Geometry check sheet. Reference: the model listing, model coordinates, mm. A direction names the side the tool comes from. Coordinates: 2 decimals unless noted, no trailing zeros. Write each loop counter-clockwise with the first axis right and the second up, starting at its lowest first coordinate (ties: lowest second). Pieces come first, ordered by that corner, then holes. Notation, with made-up numbers: (45, 76.25) -> (70, 76.25) arc R7 cw to (70, 86.25) -> close; hole circle Ø7 at (-33.75, -22.75). An arc over 180 degrees is marked (long way). Answer in a Markdown table with one row per item. Add a question column.
1. Cross-section at A-A on x = -64. Record the cut outline in (y, z).
2. Cross-section at D-D on x = 0. Record the cut outline in (y, z), and give its area (3 significant figures).
3. Depth check by flat-ended pin: P1, Ø2, axis at x = 3.5, z = -30.5, coming from the +Y side; P2, Ø15.5, axis at y = 13.5, z = -12.5, coming from the +X side; P3, Ø25, axis at y = 18, z = 13.5, coming from the -X side. Enter the tip coordinate at first touch or a pass-through.
4. Mould release check, pull along Z, two halves, no side actions. Record for faces 5 (the cylindrical face through (-64, 38, 27)), 6 (the flat face through (0, -16, 59.5)), 7 (the cylindrical face through (49.783, 37.147, -0.7)): pulls with the +Z half, pulls with the -Z half, needs draft (parallel to the pull), parting line crosses it, or undercut.
5. Scan lines: L1, parallel to X at y = 34, z = -49; L2, parallel to X at y = 37.55, z = -30; L3, parallel to X at y = 37.65, z = -30. Record each from-to range of solid material in increasing order. Write a range as from..to.
6. Cross-section at C-C on y = 31.5. Record the cut outline in (x, z).
7. Cross-section at B-B on z = -30. Record the cut outline in (x, y), and give its area (3 significant figures).
8. Set-up check for faces 1 (the flat face through (48.5, 19, 1)), 2 (the flat face through (0, -16, 58)), 3 (the flat face through (-50, 18, -1)), 4 (the flat face through (10, -9.2, 58.2)): record each of +Z, -Z, +X, -X, +Y, -Y from which the full face is reachable in a straight line by a thin tool's end or side.
```python
from build123d import *

# Parameters (mm, degrees)
SKETCH1_R                      = 5
BASE_FLANGE1_DEPTH             = 1.5
EDGE_FLANGE1_STRIP_W           = 12
EDGE_FLANGE1_STRIP_H           = 1.5
EDGE_FLANGE1_STRIP_CUT_DEPTH   = 100
EDGE_FLANGE1_STRIP_2_W         = 12
EDGE_FLANGE1_STRIP_2_H         = 1.5
EDGE_FLANGE1_STRIP_CUT_2_DEPTH = 100
EDGE_FLANGE1_DEPTH             = 100
EDGE_FLANGE1_BEND_DEPTH        = 100
EDGE_FLANGE2_STRIP_W           = 12
EDGE_FLANGE2_STRIP_H           = 1.5
EDGE_FLANGE2_STRIP_CUT_DEPTH   = 100
EDGE_FLANGE2_STRIP_2_W         = 12
EDGE_FLANGE2_STRIP_2_H         = 1.5
EDGE_FLANGE2_STRIP_CUT_2_DEPTH = 100
EDGE_FLANGE2_DEPTH             = 100
EDGE_FLANGE2_BEND_DEPTH        = 100
SKETCHED_START                 = 58.9178
SKETCHED_BEND1_OUTLINE_W       = 20
SKETCHED_BEND1_OUTLINE_H       = 1.5
SKETCHED_BEND1_DEPTH           = 32.0822
SKETCHED_START_2               = 56.266894772
SKETCHED_BEND1_2_OUTLINE_R     = 5
SKETCHED_BEND1_2_DEPTH         = 3.233105228
SKETCHED_START_3               = -10
SKETCHED_BEND1_3_DEPTH         = 20
SKETCHED_BEND1_4_DEPTH         = 20
SKETCH21_R                     = 3
CUT_EXTRUDE1_DEPTH             = 10


with BuildPart() as part:
    # Base-Flange1: sheet metal written as solids
    # Sketch1 → Base-Flange1 (new body)
    with BuildSketch(Plane(origin=(0, 0, 0), x_dir=(1, 0, 0), z_dir=(0, 1, 0))):
        with BuildLine():
            Line((10, 50), (10, 80))
            ThreePointArc((10, 80), (0, 90), (-10, 80))
            Line((-10, 80), (-10, 50))
            Line((-10, 50), (-50, 50))
            Line((-50, 50), (-50, -50))
            Line((-50, -50), (-10, -50))
            Line((-10, -50), (-10, -80))
            ThreePointArc((-10, -80), (0, -90), (10, -80))
            Line((10, -80), (10, -50))
            Line((10, -50), (50, -50))
            Line((50, -50), (50, 50))
            Line((50, 50), (10, 50))
        make_face()
        with Locations(Location((0, 80, 0), (0, 0, 270))):
            Circle(SKETCH1_R, mode=Mode.SUBTRACT)
        with Locations(Location((0, -80, 0), (0, 0, 270))):
            Circle(SKETCH1_R, mode=Mode.SUBTRACT)
    extrude(amount=-BASE_FLANGE1_DEPTH)

    # Edge-Flange1: sheet metal written as solids
    # Edge-Flange1 strip (on a plane across the edge) → Edge-Flange1 strip cut (cut)
    with BuildSketch(Plane(origin=(-50, 0, -50), x_dir=(1, 0, 0), z_dir=(0, 0, 1))):
        with Locations((-1.5, -0.75)):
            Rectangle(EDGE_FLANGE1_STRIP_W, EDGE_FLANGE1_STRIP_H)
    extrude(amount=EDGE_FLANGE1_STRIP_CUT_DEPTH, mode=Mode.SUBTRACT)

    # Edge-Flange1 strip 2 (on a plane across the edge) → Edge-Flange1 strip cut 2 (cut)
    with BuildSketch(Plane(origin=(50, 0, 50), x_dir=(-1, 0, 0), z_dir=(0, 0, -1))):
        with Locations((-1.5, -0.75)):
            Rectangle(EDGE_FLANGE1_STRIP_2_W, EDGE_FLANGE1_STRIP_2_H)
    extrude(amount=EDGE_FLANGE1_STRIP_CUT_2_DEPTH, mode=Mode.SUBTRACT)

    # Edge-Flange1 section (on a plane across the edge) → Edge-Flange1 (add)
    with BuildSketch(Plane(origin=(-50, 0, -50), x_dir=(1, 0, 0), z_dir=(0, 0, 1))):
        with BuildLine():
            Line((0, 3), (0, 38.5))
            Line((0, 38.5), (1.5, 38.5))
            Line((1.5, 38.5), (1.5, 3))
            ThreePointArc((1.5, 3), (2.378679656, 0.878679656), (4.5, 0))
            Line((4.5, 0), (4.5, -1.5))
            ThreePointArc((4.5, -1.5), (1.318019485, -0.181980515), (0, 3))
        make_face()
    extrude(amount=EDGE_FLANGE1_DEPTH)

    # Edge-Flange1 section 2 (on a plane across the edge) → Edge-Flange1 bend (add)
    with BuildSketch(Plane(origin=(50, 0, 50), x_dir=(-1, 0, 0), z_dir=(0, 0, -1))):
        with BuildLine():
            Line((0, 3), (0, 38.5))
            Line((0, 38.5), (1.5, 38.5))
            Line((1.5, 38.5), (1.5, 3))
            ThreePointArc((1.5, 3), (2.378679656, 0.878679656), (4.5, 0))
            Line((4.5, 0), (4.5, -1.5))
            ThreePointArc((4.5, -1.5), (1.318019485, -0.181980515), (0, 3))
        make_face()
    extrude(amount=EDGE_FLANGE1_BEND_DEPTH)

    # Edge-Flange2: sheet metal written as solids
    # Edge-Flange2 strip (on a plane across the edge) → Edge-Flange2 strip cut (cut)
    with BuildSketch(Plane(origin=(-50, 38.5, 50), x_dir=(0, -1, 0), z_dir=(0, 0, -1))):
        with Locations((-1.5, -0.75)):
            Rectangle(EDGE_FLANGE2_STRIP_W, EDGE_FLANGE2_STRIP_H)
    extrude(amount=EDGE_FLANGE2_STRIP_CUT_DEPTH, mode=Mode.SUBTRACT)

    # Edge-Flange2 strip 2 (on a plane across the edge) → Edge-Flange2 strip cut 2 (cut)
    with BuildSketch(Plane(origin=(50, 38.5, -50), x_dir=(0, -1, 0), z_dir=(0, 0, 1))):
        with Locations((-1.5, -0.75)):
            Rectangle(EDGE_FLANGE2_STRIP_2_W, EDGE_FLANGE2_STRIP_2_H)
    extrude(amount=EDGE_FLANGE2_STRIP_CUT_2_DEPTH, mode=Mode.SUBTRACT)

    # Edge-Flange2 section (on a plane across the edge) → Edge-Flange2 (add)
    with BuildSketch(Plane(origin=(-50, 38.5, 50), x_dir=(0, -1, 0), z_dir=(0, 0, -1))):
        with BuildLine():
            Line((0, 3), (0, 25))
            Line((0, 25), (1.5, 25))
            Line((1.5, 25), (1.5, 3))
            ThreePointArc((1.5, 3), (2.378679656, 0.878679656), (4.5, 0))
            Line((4.5, 0), (4.5, -1.5))
            ThreePointArc((4.5, -1.5), (1.318019485, -0.181980515), (0, 3))
        make_face()
    extrude(amount=EDGE_FLANGE2_DEPTH)

    # Edge-Flange2 section 2 (on a plane across the edge) → Edge-Flange2 bend (add)
    with BuildSketch(Plane(origin=(50, 38.5, -50), x_dir=(0, -1, 0), z_dir=(0, 0, 1))):
        with BuildLine():
            Line((0, 3), (0, 25))
            Line((0, 25), (1.5, 25))
            Line((1.5, 25), (1.5, 3))
            ThreePointArc((1.5, 3), (2.378679656, 0.878679656), (4.5, 0))
            Line((4.5, 0), (4.5, -1.5))
            ThreePointArc((4.5, -1.5), (1.318019485, -0.181980515), (0, 3))
        make_face()
    extrude(amount=EDGE_FLANGE2_BEND_DEPTH)

    # Sketched Bend1: read off the stored shape, not the designer's step
    # Sketched Bend1 outline → Sketched Bend1 (cut)
    with BuildSketch(Plane.XY.offset(SKETCHED_START)):
        with Locations((0, -0.75)):
            Rectangle(SKETCHED_BEND1_OUTLINE_W, SKETCHED_BEND1_OUTLINE_H)
    extrude(amount=SKETCHED_BEND1_DEPTH, mode=Mode.SUBTRACT)

    # Sketched Bend1 2 outline → Sketched Bend1 2 (add)
    with BuildSketch(Plane.XY.offset(SKETCHED_START_2)):
        with BuildLine():
            Line((10, -23.609513775), (10, -1.5))
            Line((10, -1.5), (-10, -1.5))
            Line((-10, -1.5), (-10, -23.609513775))
            ThreePointArc((-10, -23.609513775), (0, -33.609513775), (10, -23.609513775))
        make_face()
        with Locations((0, -23.609513775)):
            Circle(SKETCHED_BEND1_2_OUTLINE_R, mode=Mode.SUBTRACT)
    extrude(amount=SKETCHED_BEND1_2_DEPTH)

    # Sketched Bend1 3 outline → Sketched Bend1 3 (cut)
    with BuildSketch(Plane.YZ.offset(SKETCHED_START_3)):
        with BuildLine():
            ThreePointArc((-1.780629183, 56.266894772), (-2.887654552, 57.529889753), (-4.5, 58))
            Line((-4.5, 58), (-35, 58))
            Line((-35, 58), (-35, 56.266894772))
            Line((-35, 56.266894772), (-1.780629183, 56.266894772))
        make_face()
        with BuildLine():
            Line((1, 54), (1, 58.9178))
            Line((1, 58.9178), (-1.5, 58.9178))
            Line((-1.5, 58.9178), (-1.5, 61))
            Line((-1.5, 61), (-35, 61))
            Line((-35, 61), (-35, 59.500000008))
            Line((-35, 59.500000008), (-4.5, 59.5))
            ThreePointArc((-4.5, 59.5), (-1.318019485, 58.181980515), (0, 55))
            Line((0, 55), (0, 54))
            Line((0, 54), (1, 54))
        make_face()
    extrude(amount=SKETCHED_BEND1_3_DEPTH, mode=Mode.SUBTRACT)

    # Sketched Bend1 4 outline → Sketched Bend1 4 (add)
    with BuildSketch(Plane.YZ.offset(SKETCHED_START_3)):
        with BuildLine():
            Line((-0.182016948, 56.266894772), (-1.780629183, 56.266894772))
            ThreePointArc((-1.780629183, 56.266894772), (-1.570997401, 55.6488018), (-1.5, 55))
            Line((-1.5, 55), (-1.500000001, 54))
            Line((-1.500000001, 54), (0, 54))
            Line((0, 54), (0, 55))
            ThreePointArc((0, 55), (-0.045736664, 55.639951665), (-0.182016948, 56.266894772))
        make_face()
    extrude(amount=SKETCHED_BEND1_4_DEPTH)

    # Sketch21 → Cut-Extrude1 (cut)
    with BuildSketch(Plane(origin=(0, 38.5, 0), x_dir=(1, 0, 0), z_dir=(0, 1, 0))):
        with Locations(Location((-64, 30, 0), (0, 0, 270))):
            Circle(SKETCH21_R)
        with Locations(Location((-64, -30, 0), (0, 0, 270))):
            Circle(SKETCH21_R)
        with Locations(Location((64, 30, 0), (0, 0, 270))):
            Circle(SKETCH21_R)
        with Locations(Location((64, -30, 0), (0, 0, 270))):
            Circle(SKETCH21_R)
    extrude(amount=-CUT_EXTRUDE1_DEPTH, mode=Mode.SUBTRACT)


solid = part.part
```
Results found:
| question | item | result |
|---|---|---|
| 1 | outline | (37, -50) -> (38.5, -50) -> (38.5, -33) -> (37, -33) -> close; (37, -27) -> (38.5, -27) -> (38.5, 27) -> (37, 27) -> close; (37, 33) -> (38.5, 33) -> (38.5, 50) -> (37, 50) -> close |
| 2 | outline | (-33.61, 58) -> (-28.61, 58) -> (-28.61, 59.5) -> (-33.61, 59.5) -> close; (-18.61, 58) -> (-4.5, 58) arc R3 cw to (-1.5, 55) -> (-1.5, -75) -> (0, -75) -> (0, 55) arc R4.5 ccw to (-4.5, 59.5) -> (-18.61, 59.5) -> close; (-1.5, -90) -> (0, -90) -> (0, -85) -> (-1.5, -85) -> close |
| 2 | area | 240 mm^2 |
| 3 | P1 | stops at y = 0 |
| 3 | P2 | stops at x = 50 |
| 3 | P3 | stops at x = -50 |
| 4 | face 5 | undercut |
| 4 | face 6 | pulls with the +Z half |
| 4 | face 7 | needs draft |
| 5 | L1 | x = -50..-48.5, 48.5..50 |
| 5 | L2 | x = -75..-67, -61..-50.23, 50.23..61, 67..75 |
| 5 | L3 | x = -75..-67, -61..-50.37, 50.37..61, 67..75 |
| 6 | outline | (-50, -50) -> (-48.5, -50) -> (-48.5, 50) -> (-50, 50) -> close; (48.5, -50) -> (50, -50) -> (50, 50) -> (48.5, 50) -> close |
| 7 | outline | (-75, 37) -> (-67, 37) -> (-67, 38.5) -> (-75, 38.5) -> close; (-61, 37) -> (-53, 37) arc R3 cw to (-50, 34) -> (-50, 3) arc R4.5 ccw to (-45.5, -1.5) -> (45.5, -1.5) arc R4.5 ccw to (50, 3) -> (50, 34) arc R3 cw to (53, 37) -> (61, 37) -> (61, 38.5) -> (53, 38.5) arc R4.5 ccw to (48.5, 34) -> (48.5, 3) arc R3 cw to (45.5, 0) -> (-45.5, 0) arc R3 cw to (-48.5, 3) -> (-48.5, 34) arc R4.5 ccw to (-53, 38.5) -> (-61, 38.5) -> close; (67, 37) -> (75, 37) -> (75, 38.5) -> (67, 38.5) -> close |
| 7 | area | 313 mm^2 |
| 8 | face 1 | +Z, -Z, +Y |
| 8 | face 2 | -Z, +X, -X, -Y |
| 8 | face 3 | +Z, -Z, -X, -Y |
| 8 | face 4 | +Z, +X, +Y, -Y |
